For this review, take the finished solid that the model builds, in its own axes (mm). A direction names the side the tool comes from. Give positions to 0.01 mm unless a question says otherwise; leave off trailing zeros. Write each loop counter-clockwise with the first axis right and the second up, starting at its lowest first coordinate (ties: lowest second). Pieces come first, ordered by that corner, then holes.
1) We need section D-D on x = 13. Give the boundary of the cut face in (y, z).
2) We need section C-C on z = 6.35. Give the boundary of the cut face in (x, y) (3 decimals), and give its area (3 significant figures).
3) We need section A-A on y = -72.5. Give the boundary of the cut face in (x, z), and give its area (3 significant figures).
4) Draft analysis for pull direction X (two halves, no side actions). For faces 3 (the face through (-12.7, -63, 6)), 4 (the face through (57.147, -120.561, 6.49)), 5 (the face through (54, -115, 12.7)), state which applies: pulls with the +X half, pulls with the -X half, needs draft (parallel to the pull), parting line crosses it, or undercut.
5) For P1, Ø1, axis at x = 52, z = 10.5, coming from the +Y side, flat-tipped, find the tip position at first contact; note if it passes through.
6) We need section B-B on y = -6.35. Give the boundary of the cut face in (x, z) (3 decimals), and give its area (3 significant figures).
7) Wall thickness on line 1 along X through (y, z) = (-22.5, 7.5); line 2 along Z through (x, y) = (-9, -6.35) (3 decimals); line 3 along Y through (x, z) = (-4.5, 6.25): over which ranges is each line inside the solid? List them lowest first.
8) Machinability: for faces 1 (the face through (107.95, -56, 6)), 2 (the face through (54, -115, 0)), which of the approach directions +Z, -Z, +X, -X, +Y, -Y give a long, thin tool a straight path to every point of the face, cutting with its end or side? Answer none if there is none.
from build123d import *

# Parameters (mm, degrees)
BOSS_EXTRUDE1_DEPTH = 12.7
CUT_EXTRUDE1_REACH  = 186.587
SKETCH2_R           = 3.175
SKETCH3_R           = 3.175
CUT_EXTRUDE2_DEPTH  = 12.7


with BuildPart() as part:
    # Sketch1 → Boss-Extrude1 (new body)
    with BuildSketch(Plane.XY):
        Polygon((0, 0), (-12.7, 0), (-12.7, -127), (120.65, -127), (120.65, 0), (107.95, 0), (107.95, -114.3), (0, -114.3), align=None)
    extrude(amount=BOSS_EXTRUDE1_DEPTH)

    # Cut-Extrude1: up to this face of the body (flat: up to its plane)
    cut_extrude1_end = Plane(part.part.faces().sort_by_distance((120.65, -63.5, 6.35))[0])
    # Sketch2 → Cut-Extrude1 (cut, up to the picked face)
    with BuildSketch(Plane.ZY.offset(12.7), mode=Mode.PRIVATE) as cut_extrude1_sk1:
        with Locations(Location((6.35, -6.35, 0), (0, 0, 270))):
            Circle(SKETCH2_R)
    cut_extrude1_tool1 = split(extrude(cut_extrude1_sk1.sketch, amount=-CUT_EXTRUDE1_REACH, mode=Mode.PRIVATE), bisect_by=cut_extrude1_end, keep=Keep.BOTH, mode=Mode.PRIVATE)
    add(cut_extrude1_tool1.solids().sort_by(Axis((-12.7, -6.35, 6.35), (1, 0, 0)))[0], mode=Mode.SUBTRACT)

    # Sketch3 → Cut-Extrude2 (cut)
    with BuildSketch(Plane(origin=(0, -114.3, 0), x_dir=(1, 0, 0), z_dir=(0, 1, 0))):
        with Locations(Location((53.975, -6.35, 0), (0, 0, 180))):
            Circle(SKETCH3_R)
    extrude(amount=-CUT_EXTRUDE2_DEPTH, mode=Mode.SUBTRACT)


solid = part.part
Results list:
1. outline: (-127, 0) - (-114.3, 0) - (-114.3, 12.7) - (-127, 12.7) - close
2. outline: (-12.7, -127) - (50.8, -127) - (50.8, -114.3) - (0, -114.3) - (0, -9.525) - (-12.7, -9.525) - close; (-12.7, -3.175) - (0, -3.175) - (0, 0) - (-12.7, 0) - close; (57.15, -127) - (120.65, -127) - (120.65, -9.525) - (107.95, -9.525) - (107.95, -114.3) - (57.15, -114.3) - close; (107.95, -3.175) - (120.65, -3.175) - (120.65, 0) - (107.95, 0) - close
2. area: 4,350 mm2
3. outline: (-12.7, 0) - (0, 0) - (0, 12.7) - (-12.7, 12.7) - close; (107.95, 0) - (120.65, 0) - (120.65, 12.7) - (107.95, 12.7) - close
3. area: 323 mm2
4. face 3: pulls with the -X half
4. face 4: undercut
4. face 5: needs draft
5. P1: stops at y = -114.3
6. outline: (-12.7, 0) - (0, 0) - (0, 3.175) - (-12.7, 3.175) - close; (-12.7, 9.525) - (0, 9.525) - (0, 12.7) - (-12.7, 12.7) - close; (107.95, 0) - (120.65, 0) - (120.65, 3.175) - (107.95, 3.175) - close; (107.95, 9.525) - (120.65, 9.525) - (120.65, 12.7) - (107.95, 12.7) - close
6. area: 161 mm2
7. line 1: x = -12.7 to 0, 107.95 to 120.65
7. line 2: z = 0 to 3.175, 9.525 to 12.7
7. line 3: y = -127 to -9.52, -3.18 to 0
8. face 1: +Z, -Z, +Y
8. face 2: -Z, +X, -X, +Y, -Y
